Verification items for the finished model (mm, model axes). A direction names the side the tool comes from. Round coordinates to 2 decimals unless told otherwise and drop trailing zeros. Loops run counter-clockwise (first coordinate to the right, second up) from the corner with the lowest first, then second, coordinate; pieces in that order, holes last.
from build123d import *

# Parameters (mm, degrees)
SKETCH_1_R          = 2.1
SKETCH_1_R_2        = 1.6
SKETCH_1_R_3        = 11
SKETCH_1_R_4        = 2.5
EXTRUDE_1_DEPTH     = 5
SKETCH_2_R          = 3.689501017
SKETCH_2_R_2        = 3.294011366
EXTRUDE_2_DEPTH     = 5
CUT_EXTRUDE_1_REACH = 156.458
SKETCH_3_R          = 2
SKETCH_5_W          = 25.495020877
SKETCH_5_H          = 33.419148988
EXTRUDE_3_DEPTH     = 5
CUT_EXTRUDE_2_REACH = 156.458
SKETCH_4_R          = 2
FILLET_1_R          = 4
CUT_EXTRUDE_3_DEPTH = 10


with BuildPart() as part:
    # Sketch 1 → Extrude 1 (new body)
    with BuildSketch(Plane(origin=(0, 0, 0), x_dir=(-1, 0, 0), z_dir=(0, 0, -1))):
        with BuildLine():
            Line((-26.5, -36.5), (26.5, -36.5))
            ThreePointArc((26.5, -36.5), (31.295831523, -35.274964387), (34.916650165, -31.9))
            ThreePointArc((34.916650165, -31.9), (40.347878128, -26.837553419), (47.541625413, -25))
            Line((47.541625413, -25), (150, -25))
            Line((150, -25), (150, 25))
            Line((150, 25), (47.541625413, 25))
            ThreePointArc((47.541625413, 25), (40.347878128, 26.837553419), (34.916650165, 31.9))
            ThreePointArc((34.916650165, 31.9), (31.295831523, 35.274964387), (26.5, 36.5))
            Line((26.5, 36.5), (-26.5, 36.5))
            ThreePointArc((-26.5, 36.5), (-31.295831523, 35.274964387), (-34.916650165, 31.9))
            ThreePointArc((-34.916650165, 31.9), (-40.347878128, 26.837553419), (-47.541625413, 25))
            Line((-47.541625413, 25), (-150, 25))
            Line((-150, 25), (-150, -25))
            Line((-150, -25), (-47.541625413, -25))
            ThreePointArc((-47.541625413, -25), (-40.347878128, -26.837553419), (-34.916650165, -31.9))
            ThreePointArc((-34.916650165, -31.9), (-31.295831523, -35.274964387), (-26.5, -36.5))
        make_face()
        with Locations(Location((-29, 29, 0), (0, 0, 180))):
            Circle(SKETCH_1_R, mode=Mode.SUBTRACT)
        with Locations(Location((-29, -29, 0), (0, 0, 180))):
            Circle(SKETCH_1_R, mode=Mode.SUBTRACT)
        with Locations(Location((29, -29, 0), (0, 0, 180))):
            Circle(SKETCH_1_R, mode=Mode.SUBTRACT)
        with Locations(Location((29, 29, 0), (0, 0, 180))):
            Circle(SKETCH_1_R, mode=Mode.SUBTRACT)
        with Locations(Location((-54.5, 0, 0), (0, 0, 180))):
            Circle(SKETCH_1_R, mode=Mode.SUBTRACT)
        with Locations(Location((-114, 0, 0), (0, 0, 180))):
            Circle(SKETCH_1_R_2, mode=Mode.SUBTRACT)
        with Locations(Location((-5.303300859, 5.303300859, 0), (0, 0, 180))):
            Circle(SKETCH_1_R_2, mode=Mode.SUBTRACT)
        with Locations(Location((5.303300859, 5.303300859, 0), (0, 0, 180))):
            Circle(SKETCH_1_R_2, mode=Mode.SUBTRACT)
        with Locations(Location((70, 0, 0), (0, 0, 180))):
            Circle(SKETCH_1_R_3, mode=Mode.SUBTRACT)
        with Locations(Location((-85.5, 0, 0), (0, 0, 180))):
            Circle(SKETCH_1_R, mode=Mode.SUBTRACT)
        with Locations(Location((85.5, 0, 0), (0, 0, 180))):
            Circle(SKETCH_1_R, mode=Mode.SUBTRACT)
        with Locations(Location((54.5, 0, 0), (0, 0, 180))):
            Circle(SKETCH_1_R, mode=Mode.SUBTRACT)
        with Locations(Location((-70, 0, 0), (0, 0, 180))):
            Circle(SKETCH_1_R_3, mode=Mode.SUBTRACT)
        with Locations(Location((5.303300859, -5.303300859, 0), (0, 0, 180))):
            Circle(SKETCH_1_R_2, mode=Mode.SUBTRACT)
        with Locations(Location((-5.303300859, -5.303300859, 0), (0, 0, 180))):
            Circle(SKETCH_1_R_2, mode=Mode.SUBTRACT)
        with Locations(Location((114, 0, 0), (0, 0, 180))):
            Circle(SKETCH_1_R_2, mode=Mode.SUBTRACT)
        with Locations(Location((146, 0, 0), (0, 0, 180))):
            Circle(SKETCH_1_R_2, mode=Mode.SUBTRACT)
        with Locations(Location((130, 22, 0), (0, 0, 180))):
            Circle(SKETCH_1_R_2, mode=Mode.SUBTRACT)
        with Locations(Location((130, -22, 0), (0, 0, 180))):
            Circle(SKETCH_1_R_2, mode=Mode.SUBTRACT)
        with Locations(Location((-130, -22, 0), (0, 0, 180))):
            Circle(SKETCH_1_R_2, mode=Mode.SUBTRACT)
        with Locations(Location((-130, 22, 0), (0, 0, 180))):
            Circle(SKETCH_1_R_2, mode=Mode.SUBTRACT)
        with Locations(Location((-146, 0, 0), (0, 0, 180))):
            Circle(SKETCH_1_R_2, mode=Mode.SUBTRACT)
        with Locations(Location((100, 15, 0), (0, 0, 180))):
            Circle(SKETCH_1_R_4, mode=Mode.SUBTRACT)
        with Locations(Location((-100, 15, 0), (0, 0, 180))):
            Circle(SKETCH_1_R_4, mode=Mode.SUBTRACT)
        with Locations(Location((-100, -15, 0), (0, 0, 180))):
            Circle(SKETCH_1_R_4, mode=Mode.SUBTRACT)
        with Locations(Location((100, -15, 0), (0, 0, 180))):
            Circle(SKETCH_1_R_4, mode=Mode.SUBTRACT)
    extrude(amount=-EXTRUDE_1_DEPTH)

    # Sketch 2 → Extrude 2 (add)
    with BuildSketch(Plane.XY.offset(5)):
        with Locations((-85.5, 0)):
            Circle(SKETCH_2_R)
        with Locations((-54.5, 0)):
            Circle(SKETCH_2_R_2)
    extrude_2 = extrude(amount=-EXTRUDE_2_DEPTH)

    # Sketch 3 → Cut-Extrude 1 (cut, up to next)
    with BuildSketch(Plane.XY.offset(5), mode=Mode.PRIVATE) as cut_extrude_1_sk1:
        with Locations((-85, 0)):
            Circle(SKETCH_3_R)
    cut_extrude_1_tool1 = extrude(cut_extrude_1_sk1.sketch, amount=-CUT_EXTRUDE_1_REACH, mode=Mode.PRIVATE) & part.part
    # Sketch 3 → Cut-Extrude 1 (cut, up to next)
    with BuildSketch(Plane.XY.offset(5), mode=Mode.PRIVATE) as cut_extrude_1_sk2:
        with Locations((-55, 0)):
            Circle(SKETCH_3_R)
    cut_extrude_1_tool2 = extrude(cut_extrude_1_sk2.sketch, amount=-CUT_EXTRUDE_1_REACH, mode=Mode.PRIVATE) & part.part
    cut_extrude_1_1 = cut_extrude_1_tool1.solids().sort_by_distance((-85, 0, 5))[0]
    add(cut_extrude_1_1, mode=Mode.SUBTRACT)
    cut_extrude_1_2 = cut_extrude_1_tool2.solids().sort_by_distance((-55, 0, 5))[0]
    add(cut_extrude_1_2, mode=Mode.SUBTRACT)
    cut_extrude_1 = cut_extrude_1_1 + cut_extrude_1_2  # Cut-Extrude 1 as one shape, for the pattern or mirror that repeats it

    # Mirror 1: Extrude 2, Cut-Extrude 1 across plane
    add(extrude_2.mirror(Plane.ZY))
    add(cut_extrude_1.mirror(Plane.ZY), mode=Mode.SUBTRACT)

    # Sketch 5 → Extrude 3 (add)
    with BuildSketch(Plane(origin=(0, 0, 0), x_dir=(-1, 0, 0), z_dir=(0, 0, -1))):
        Polygon((47.541625413, 25), (47.541625413, 36.5), (21.518894716, 36.5), (-47.541625413, 36.5), (-47.541625413, 25), (-47.541625413, -25), (-47.541625413, -36.5), (26.5, -36.5), (47.541625413, -36.5), (47.541625413, -25), align=None)
        with Locations((-1.313647453, -0.287111202)):
            Rectangle(SKETCH_5_W, SKETCH_5_H, mode=Mode.SUBTRACT)
    extrude(amount=-EXTRUDE_3_DEPTH)

    # Sketch 4 → Cut-Extrude 2 (cut, up to next)
    with BuildSketch(Plane(origin=(0, 0, 0), x_dir=(-1, 0, 0), z_dir=(0, 0, -1)), mode=Mode.PRIVATE) as cut_extrude_2_sk1:
        with Locations((28.991378029, -28.991378029)):
            Circle(SKETCH_4_R)
    cut_extrude_2_tool1 = extrude(cut_extrude_2_sk1.sketch, amount=-CUT_EXTRUDE_2_REACH, mode=Mode.PRIVATE) & part.part
    # Sketch 4 → Cut-Extrude 2 (cut, up to next)
    with BuildSketch(Plane(origin=(0, 0, 0), x_dir=(-1, 0, 0), z_dir=(0, 0, -1)), mode=Mode.PRIVATE) as cut_extrude_2_sk2:
        with Locations((-28.991378029, 28.991378029)):
            Circle(SKETCH_4_R)
    cut_extrude_2_tool2 = extrude(cut_extrude_2_sk2.sketch, amount=-CUT_EXTRUDE_2_REACH, mode=Mode.PRIVATE) & part.part
    # Sketch 4 → Cut-Extrude 2 (cut, up to next)
    with BuildSketch(Plane(origin=(0, 0, 0), x_dir=(-1, 0, 0), z_dir=(0, 0, -1)), mode=Mode.PRIVATE) as cut_extrude_2_sk3:
        with Locations((28.991378029, 28.991378029)):
            Circle(SKETCH_4_R)
    cut_extrude_2_tool3 = extrude(cut_extrude_2_sk3.sketch, amount=-CUT_EXTRUDE_2_REACH, mode=Mode.PRIVATE) & part.part
    # Sketch 4 → Cut-Extrude 2 (cut, up to next)
    with BuildSketch(Plane(origin=(0, 0, 0), x_dir=(-1, 0, 0), z_dir=(0, 0, -1)), mode=Mode.PRIVATE) as cut_extrude_2_sk4:
        with Locations((-28.991378029, -28.991378029)):
            Circle(SKETCH_4_R)
    cut_extrude_2_tool4 = extrude(cut_extrude_2_sk4.sketch, amount=-CUT_EXTRUDE_2_REACH, mode=Mode.PRIVATE) & part.part
    add(cut_extrude_2_tool1.solids().sort_by_distance((-28.991378, -28.991378, 0))[0], mode=Mode.SUBTRACT)
    add(cut_extrude_2_tool2.solids().sort_by_distance((28.991378, 28.991378, 0))[0], mode=Mode.SUBTRACT)
    add(cut_extrude_2_tool3.solids().sort_by_distance((-28.991378, 28.991378, 0))[0], mode=Mode.SUBTRACT)
    add(cut_extrude_2_tool4.solids().sort_by_distance((28.991378, -28.991378, 0))[0], mode=Mode.SUBTRACT)

    # Fillet 1
    fillet_1_edges = [part.edges().sort_by_distance(p)[0] for p in [
        (-47.541625413, 36.5, 2.5),
        (47.541625413, -36.5, 2.5),
        (47.541625413, -25, 2.5),
        (47.541625413, 25, 2.5),
        (-47.541625413, 25, 2.5),
        (-47.541625413, -36.5, 2.5),
        (47.541625413, 36.5, 2.5),
        (-47.541625413, -25, 2.5),
    ]]
    fillet(fillet_1_edges, radius=FILLET_1_R)

    # Sketch 6 → Cut-Extrude 3 (cut)
    with BuildSketch(Plane(origin=(0, 0, 0), x_dir=(-1, 0, 0), z_dir=(0, 0, -1))):
        with BuildLine():
            Line((-21.414213562, 19.085786438), (-39.085786438, 1.414213562))
            ThreePointArc((-39.085786438, 1.414213562), (-39.671572875, 0), (-39.085786438, -1.414213562))
            Line((-39.085786438, -1.414213562), (-21.414213562, -19.085786438))
            ThreePointArc((-21.414213562, -19.085786438), (-19.234633135, -19.51933194), (-18, -17.671572875))
            Line((-18, -17.671572875), (-18, 17.671572875))
            ThreePointArc((-18, 17.671572875), (-19.234633135, 19.51933194), (-21.414213562, 19.085786438))
        make_face()
        with BuildLine():
            Line((18, -17.671572875), (18, 17.671572875))
            ThreePointArc((18, 17.671572875), (19.234633135, 19.51933194), (21.414213562, 19.085786438))
            Line((21.414213562, 19.085786438), (39.085786438, 1.414213562))
            ThreePointArc((39.085786438, 1.414213562), (39.671572875, 0), (39.085786438, -1.414213562))
            Line((39.085786438, -1.414213562), (21.414213562, -19.085786438))
            ThreePointArc((21.414213562, -19.085786438), (19.234633135, -19.51933194), (18, -17.671572875))
        make_face()
    extrude(amount=-CUT_EXTRUDE_3_DEPTH, mode=Mode.SUBTRACT)


solid = part.part
1. Gauge pin test, flat ends, axial feed: P1, Ø2.5, axis at x = -28.99, y = -28.99, coming from the -Z side; P2, Ø1.5, axis at x = 103.5, z = 2.5, coming from the +Y side; P3, Ø6.5, axis at x = 28.99, y = 28.99, coming from the +Z side; P4, Ø1.8, axis at y = 31.5, z = 2.5, coming from the +X side. Record the tip position at first contact, or that the pin passes through.
2. Release check for a two-part mould opening along X. For faces 1 (the face through (-150, 0, 2)), 2 (the face through (-18, 0, 2)), 3 (the face through (101, -25, 2)) record: released by +X, released by -X, zero draft, split by the parting line, or undercut.
3. Section check A-A (x = 70). Enter the section's corners in (y, z), then the cut area to 3 significant figures.
4. Scan lines: L1, parallel to X at y = -22, z = 3.1; L2, parallel to Y at x = 100, z = 1; L3, parallel to X at y = -30, z = 3.7. Record each from-to range of solid material in increasing order.
5. Tool access check on faces 4 (the face through (150, 0, 2)), 5 (the face through (100, 25, 2)), 6 (the face through (18, 0, 2)). Record the directions out of +Z, -Z, +X, -X, +Y, -Y that give a thin tool (end or side, any length) a straight path to the whole face; none if there is none.
6. Section check B-B (z = 2.5). Give the number of separate pieces and of enclosed holes in the cut face, then the cut area to 3 significant figures.
Taken from the geometry:
1. P1: passes through
1. P2: stops at y = 25
1. P3: stops at z = 5
1. P4: stops at x = 47.54
2. face 1: released by -X
2. face 2: undercut
2. face 3: zero draft
3. outline: (-25, 0) - (-11, 0) - (-11, 5) - (-25, 5) - close; (11, 0) - (25, 0) - (25, 5) - (11, 5) - close
3. area: 140 mm2
4. L1: x = -150 to -131.6, -128.4 to 128.4, 131.6 to 150
4. L2: y = -25 to -17.5, -12.5 to 12.5, 17.5 to 25
4. L3: x = -47.54 to -30.72, -27.26 to 27.26, 30.72 to 47.54
5. face 4: +Z, -Z, +X, +Y, -Y
5. face 5: +Z, -Z, +X, +Y
5. face 6: +Z, -Z
6. separate pieces: 1
6. enclosed holes: 28
6. area: 15,200 mm2
